Verification items for the finished model (mm, model axes). Face numbers are marked on the shaded views. A direction names the side the tool comes from. Coordinates: 2 decimals unless noted, no trailing zeros. Write each loop counter-clockwise with the first axis right and the second up, starting at its lowest first coordinate (ties: lowest second). Pieces come first, ordered by that corner, then holes. Notation, with made-up numbers: (-23, -24) -> (-11, -24) arc R19 cw to (-11, 0) -> close; hole circle Ø3 at (67, 81). An arc over 180 degrees is marked (long way). Use CSV: the item, a comma, the result in double quotes.
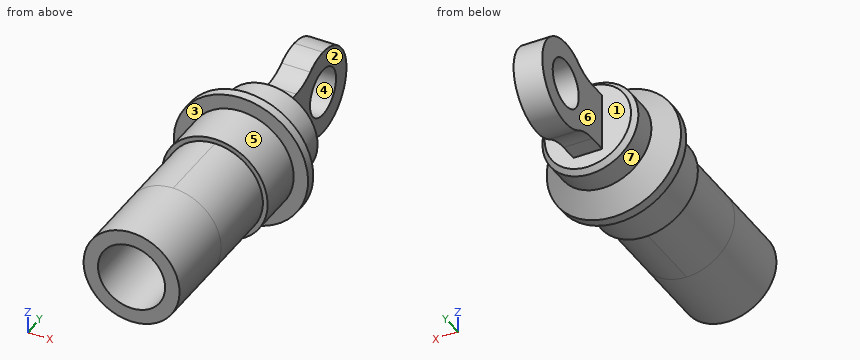
```python
from build123d import *

# Parameters (mm, degrees)
SKETCH1_R            = 5
BOSS_EXTRUDE1_DEPTH  = 8
SKETCH2_R            = 5.5
BOSS_EXTRUDE2_DEPTH  = 5
SKETCH3_R            = 7
BOSS_EXTRUDE3_DEPTH  = 1
CHAMFER2_SIZE        = 0.5
SKETCH48_W           = 2.996334688
SKETCH48_H           = 6
BOSS_EXTRUDE7_DEPTH  = 7
SKETCH50_R           = 4.5
BOSS_EXTRUDE9_DEPTH  = 2.99
BOSS_EXTRUDE10_START = -2.99
SKETCH51_R           = 4.5
BOSS_EXTRUDE10_DEPTH = 2.99
SKETCH52_R           = 2.5
CUT_EXTRUDE1_DEPTH   = 4
BOSS_EXTRUDE11_START = 16
SKETCH56_R           = 5
BOSS_EXTRUDE11_DEPTH = 16
SKETCH57_R           = 3.25
CUT_EXTRUDE7_DEPTH   = 21
SKETCH59_R           = 3.5
CUT_EXTRUDE10_DEPTH  = 26
FILLET1_R            = 5


with BuildPart() as part:
    # Sketch1 → Boss-Extrude1 (new body)
    with BuildSketch(Plane(origin=(0, 0, 0), x_dir=(1, 0, 0), z_dir=(0, 1, 0))):
        with Locations(Location((0, 0, 0), (0, 0, 270))):
            Circle(SKETCH1_R)
    extrude(amount=BOSS_EXTRUDE1_DEPTH)

    # Sketch2 → Boss-Extrude2 (add)
    with BuildSketch(Plane(origin=(0, 8, 0), x_dir=(1, 0, 0), z_dir=(0, 1, 0))):
        with Locations(Location((0, 0, 0), (0, 0, 270))):
            Circle(SKETCH2_R)
    extrude(amount=BOSS_EXTRUDE2_DEPTH)

    # Sketch3 → Boss-Extrude3 (add)
    with BuildSketch(Plane(origin=(0, 13, 0), x_dir=(1, 0, 0), z_dir=(0, 1, 0))):
        with Locations(Location((0, 0, 0), (0, 0, 270))):
            Circle(SKETCH3_R)
    extrude(amount=BOSS_EXTRUDE3_DEPTH)

    # Sketch47 → Revolve1 (revolve)
    with BuildSketch(Plane(origin=(0, 0, 0), x_dir=(0, 0, -1), z_dir=(1, 0, 0))):
        Polygon((0, 14), (0, 19), (5, 19), (5, 16), (7, 14), align=None)
    revolve(axis=Axis((0, 14, 0), (0, 1, 0)))

    # Chamfer2
    chamfer2_edges = [part.edges().sort_by_distance(p)[0] for p in [
        (0, 19, 5),
    ]]
    chamfer(chamfer2_edges, length=CHAMFER2_SIZE)

    # Sketch48 → Boss-Extrude7 (add)
    with BuildSketch(Plane(origin=(0, 19, 0), x_dir=(1, 0, 0), z_dir=(0, 1, 0))):
        Rectangle(SKETCH48_W, SKETCH48_H)
    extrude(amount=BOSS_EXTRUDE7_DEPTH)

    # Sketch50 → Boss-Extrude9 (add)
    with BuildSketch(Plane(origin=(1.498167344, 0, 0), x_dir=(0, 0, -1), z_dir=(1, 0, 0))):
        with Locations((0, 26)):
            Circle(SKETCH50_R)
    extrude(amount=-BOSS_EXTRUDE9_DEPTH)

    # Sketch51 → Boss-Extrude10 (add)
    with BuildSketch(Plane.ZY.offset(1.498167344).offset(BOSS_EXTRUDE10_START)):
        with Locations((0, 26)):
            Circle(SKETCH51_R)
    extrude(amount=BOSS_EXTRUDE10_DEPTH)

    # Sketch52 → Cut-Extrude1 (cut)
    with BuildSketch(Plane.ZY.offset(1.498167344)):
        with Locations((0, 26)):
            Circle(SKETCH52_R)
    extrude(amount=-CUT_EXTRUDE1_DEPTH, mode=Mode.SUBTRACT)

    # Sketch56 → Boss-Extrude11 (add)
    with BuildSketch(Plane.XZ.offset(-8).offset(BOSS_EXTRUDE11_START)):
        with Locations(Location((0, 0, 0), (0, 0, 270))):
            Circle(SKETCH56_R)
    extrude(amount=-BOSS_EXTRUDE11_DEPTH)

    # Sketch57 → Cut-Extrude7 (cut)
    with BuildSketch(Plane.XZ.offset(8)):
        with Locations(Location((0, 0, 0), (0, 0, 270))):
            Circle(SKETCH57_R)
    extrude(amount=-CUT_EXTRUDE7_DEPTH, mode=Mode.SUBTRACT)

    # Sketch59 → Cut-Extrude10 (cut)
    with BuildSketch(Plane(origin=(0, -8, 0), x_dir=(-1, 0, 0), z_dir=(0, -1, 0))):
        with Locations(Location((0, 0, 0), (0, 0, 90))):
            Circle(SKETCH59_R)
    extrude(amount=-CUT_EXTRUDE10_DEPTH, mode=Mode.SUBTRACT)

    # Fillet1
    fillet1_edges = [part.edges().sort_by_distance(p)[0] for p in [
        (0, 22.645898034, 3),
        (0, 22.645898034, -3),
    ]]
    fillet(fillet1_edges, radius=FILLET1_R)


solid = part.part
```
1) Cross-section at C-C (y = -0.5). Record the boundary of the cut face in (x, z).
Return value:
outline,"circle Ø10 at (0, 0); hole circle Ø7 at (0, 0)"
2) Mould release check, pull along Y, two halves, no side actions. Record for the marked faces 1, 2, 3 and 4: released by +Y, released by -Y, zero draft, split by the parting line, or undercut.
Return value:
face 1,"undercut"
face 2,"zero draft"
face 3,"released by -Y"
face 4,"undercut"
3) Scan lines: L1, parallel to Z at x = -0.25, y = 0; L2, parallel to Z at x = -0.6, y = 26; L3, parallel to Y at x = -0.55, z = 0. Record each from-to range of solid material in increasing order.
Return value:
L1,"-4.99 to -3.49, 3.49 to 4.99"
L2,"-4.5 to -2.5, 2.5 to 4.5"
L3,"18 to 23.5, 28.5 to 30.5"
4) Set-up check for the marked faces 5, 6 and 7: record each of +Z, -Z, +X, -X, +Y, -Y from which the full face is reachable in a straight line by a thin tool's end or side.
Return value:
face 5,"-Y"
face 6,"+Z, -Z, -X, +Y"
face 7,"+Y"
5) Gauge pin test, flat ends, axial feed: pin 1 (1.5 mm diameter, centred on x = 2.5, z = -5, fed in from +Y); pin 2 (6 mm diameter, centred on x = -3.5, y = 16, fed in from -Z); pin 3 (5 mm diameter, centred on x = -3.5, y = 4.5, fed in from +Z). Record the tip position at first contact, or that the pin passes through.
Return value:
pin 1,"y = 18.66"
pin 2,"z = -6.88"
pin 3,"z = 4.9"
6) Cross-section at B-B (y = 24). Record the boundary of the cut face in (x, z).
Return value:
outline,"(-1.5, -4.03) -> (1.5, -4.03) -> (1.5, -1.5) -> (-1.5, -1.5) -> close; (-1.5, 1.5) -> (1.5, 1.5) -> (1.5, 4.03) -> (-1.5, 4.03) -> close"
